from build123d import *

# Parameters (mm, degrees)
ESQUISSE2_W                  = 100
ESQUISSE2_H                  = 100
BOSS_EXTRU_1_DEPTH           = 51
BOSS_EXTRU_1_TAPER           = 20
ENL_V_MAT_EXTRU_1_DEPTH      = 140.622233322
ENL_V_MAT_EXTRU_1_DEPTH_BACK = 140.622233322
ESQUISSE3_R                  = 25
ENL_V_MAT_EXTRU_2_DEPTH      = 140.622233322
ENL_V_MAT_EXTRU_2_DEPTH_BACK = 10
ESQUISSE5_R                  = 35
ENL_V_START                  = -10
ESQUISSE6_R                  = 35
ENL_V_MAT_EXTRU_3_DEPTH      = 10
ESQUISSE7_W                  = 50
ESQUISSE7_H                  = 50
ENL_V_MAT_EXTRU_4_DEPTH      = 140.622233322
CONG_1_R                     = 15
ENL_V_MAT_EXTRU_8_DEPTH      = 10
BOSS_EXTRU_2_DEPTH           = 10
CONG_2_R                     = 5


with BuildPart() as part:
    # Esquisse2 → Boss.-Extru.1 (new body)
    with BuildSketch(Plane.XY):
        with Locations((-23.410404624, -10.838150289)):
            Rectangle(ESQUISSE2_W, ESQUISSE2_H)
    boss_extru_1 = extrude(amount=BOSS_EXTRU_1_DEPTH, taper=BOSS_EXTRU_1_TAPER)

    # Symétrie4: Boss.-Extru.1 across plane
    add(boss_extru_1.mirror(Plane.XY.offset(51)))

    # Esquisse3 → Enlèv. mat.-Extru.1 (cut, two sides: drawn at the far end of the back side and taken through both)
    with BuildSketch(Plane.XY.offset(102).offset(-ENL_V_MAT_EXTRU_1_DEPTH_BACK)):
        with Locations((-23.410404624, -10.838150289)):
            Circle(ESQUISSE3_R)
    extrude(amount=ENL_V_MAT_EXTRU_1_DEPTH + ENL_V_MAT_EXTRU_1_DEPTH_BACK, mode=Mode.SUBTRACT)

    # Esquisse5 → Enlèv. mat.-Extru.2 (cut, two sides: drawn at the far end of the back side and taken through both)
    with BuildSketch(Plane.XY.offset(102).offset(-ENL_V_MAT_EXTRU_2_DEPTH_BACK)):
        with Locations(Location((-23.410404624, -10.838150289, 0), (0, 0, 180))):
            Circle(ESQUISSE5_R)
    extrude(amount=ENL_V_MAT_EXTRU_2_DEPTH + ENL_V_MAT_EXTRU_2_DEPTH_BACK, mode=Mode.SUBTRACT)

    # Esquisse6 → Enlèv. mat.-Extru.3 (cut)
    with BuildSketch(Plane(origin=(0, 0, 0), x_dir=(-1, 0, 0), z_dir=(0, 0, -1)).offset(ENL_V_START)):
        with Locations((23.410404624, -10.838150289)):
            Circle(ESQUISSE6_R)
    extrude(amount=ENL_V_MAT_EXTRU_3_DEPTH, mode=Mode.SUBTRACT)

    # Esquisse7 → Enlèv. mat.-Extru.4 (cut, through all)
    with BuildSketch(Plane(origin=(0, 0, 0), x_dir=(-1, 0, 0), z_dir=(0, 0, -1))):
        with Locations((48.410404624, -35.838150289)):
            Rectangle(ESQUISSE7_W, ESQUISSE7_H)
    extrude(amount=-ENL_V_MAT_EXTRU_4_DEPTH, mode=Mode.SUBTRACT)

    # Congé1
    cong_1_edges = [part.edges().sort_by_distance(p)[0] for p in [
        (8.027113428, -10.838150289, 51),
        (-23.410404624, 20.599367763, 51),
        (-54.847922677, 4.880608737, 51),
    ]]
    fillet(cong_1_edges, radius=CONG_1_R)

    # Esquisse8 → Enlèv. mat.-Extru.8 (cut)
    with BuildSketch(Plane(origin=(0, 0, 0), x_dir=(-1, 0, 0), z_dir=(0, 0, -1))):
        with BuildLine():
            Line((-15.12691495, 31.941809973), (-4.520313233, 21.335208255))
            ThreePointArc((-4.520313233, 21.335208255), (-4.520313233, 17.092567568), (-8.76295392, 17.092567568))
            Line((-8.76295392, 17.092567568), (-19.369555638, 27.699169286))
            ThreePointArc((-19.369555638, 27.699169286), (-19.369555638, 31.941809973), (-15.12691495, 31.941809973))
        make_face()
        with BuildLine():
            Line((-19.369555638, -49.375469864), (-8.76295392, -38.768868146))
            ThreePointArc((-8.76295392, -38.768868146), (-4.520313233, -38.768868146), (-4.520313233, -43.011508833))
            Line((-4.520313233, -43.011508833), (-15.12691495, -53.618110551))
            ThreePointArc((-15.12691495, -53.618110551), (-19.369555638, -53.618110551), (-19.369555638, -49.375469864))
        make_face()
        with BuildLine():
            Line((51.341122481, 21.335208255), (61.947724199, 31.941809973))
            ThreePointArc((61.947724199, 31.941809973), (66.190364886, 31.941809973), (66.190364886, 27.699169286))
            Line((66.190364886, 27.699169286), (55.583763168, 17.092567568))
            ThreePointArc((55.583763168, 17.092567568), (51.341122481, 17.092567568), (51.341122481, 21.335208255))
        make_face()
    extrude(amount=-ENL_V_MAT_EXTRU_8_DEPTH, mode=Mode.SUBTRACT)

    # Esquisse9 → Boss.-Extru.2 (add)
    with BuildSketch(Plane(origin=(0, 0, 0), x_dir=(-1, 0, 0), z_dir=(0, 0, -1))):
        Polygon((-26.589595376, -60.838150289), (23.410404624, -60.838150289), (23.410404624, -57.838150289), (-23.589595376, -57.838150289), (-23.589595376, 36.161849711), (70.410404624, 36.161849711), (70.410404624, -10.838150289), (73.410404624, -10.838150289), (73.410404624, 39.161849711), (-26.589595376, 39.161849711), align=None)
    extrude(amount=BOSS_EXTRU_2_DEPTH)

    # Congé2
    cong_2_edges = [part.edges().sort_by_distance(p)[0] for p in [
        (-23.410404624, 39.161849711, 0),
        (26.589595376, -10.838150289, 0),
        (-73.410404624, 14.161849711, 0),
        (1.589595376, -60.838150289, 0),
    ]]
    fillet(cong_2_edges, radius=CONG_2_R)


solid = part.part
Part model, mm, in its own coordinate system. A direction names the side the tool comes from. Round coordinates to 2 decimals unless told otherwise and drop trailing zeros. Write each loop counter-clockwise with the first axis right and the second up, starting at its lowest first coordinate (ties: lowest second). Pieces come first, ordered by that corner, then holes. Notation, with made-up numbers: M 59.5,12 L 116.5,12 A6 cw 116.5,21 Z; hole C 59.25,33 d1. An arc over 180 degrees is marked long. Return JSON: item names as keys, results as strings. Group by question number.
(1) Pin check, flat tips, straight feed: pin 1 Ø18.5 at (x, y) = (-58.5, 25) entering from -Z; pin 2 Ø5 at (y, z) = (-29, 2) entering from +X (3 decimals); pin 3 Ø2 at (y, z) = (8.5, 85.5) entering from +X. Stop position of each tip, or through.
(2) Saw through at A-A on y = -51. Write the cut outline in (x, z), then the cut area to 3 significant figures.
(3) Saw through at C-C on z = 8.5. Write the cut outline in (x, y).
(4) Two-plate mould, pull along X, no slides. Class faces 1 (the face through (-5.16, 6.25, 50.43)), 2 (the face through (18.36, -10.14, 79.39)), 3 (the face through (-24.11, 30.78, 23.03)): +X half, -X half, draft (parallel to the pull), parting line (faces both ways), or undercut.
(5) Which spindle directions (+Z, -Z, +X, -X, +Y, -Y) get a long thin tool onto all of the face, cutting with end or side? Do faces 4 (the face through (-70.41, 13, -5)), 5 (the face through (14.141, -44.146, 4.93)), 6 (the face through (-65.18, 8.26, 79.39)), 7 (the face through (-24.11, 30.931, 79.386)). Say none if no direction does.
(6) Drill centre lines: probe 1 along Z at (x, y) = (-40, 10); probe 2 along X at (y, z) = (5, 36); probe 3 along Y at (x, z) = (-31.5, -2.5). Where is each one in solid material? Low to high.
(7) Saw through at B-B on x = -10. Write the cut outline in (y, z).
Returned:
{
 "1": {"pin 1": "z = 0", "pin 2": "x = 26.575", "pin 3": "x = 20.95"},
 "2": {"outline": "M -23.41,0 L 12.51,0 L 12.51,10 L 20.21,10 L 20.21,0 L 23.59,0 L 23.59,-10 L 26.59,-10 L 26.59,-0.88 A5 ccw 26.29,0.83 L 16.75,27.03 L -23.41,27.03 Z; M -23.41,74.97 L 16.75,74.97 L 26.59,102 L -23.41,102 Z", "area": "2,390 mm²"},
 "3": {"outline": "M -70.32,-10.84 L -58.41,-10.84 A35 cw long -23.41,-45.84 L -23.41,-57.74 L 23.5,-57.74 L 23.5,36.07 L -70.32,36.07 Z; hole M -66.19,27.7 L -55.58,17.09 A3 ccw -51.34,21.34 L -61.95,31.94 A3 ccw Z; hole M 4.52,-43.01 L 15.13,-53.62 A3 ccw 19.37,-49.38 L 8.76,-38.77 A3 ccw Z; hole M 4.52,21.34 A3 ccw 8.76,17.09 L 19.37,27.7 A3 ccw 15.13,31.94 Z"},
 "4": {"face 1": "undercut", "face 2": "+X half", "face 3": "draft"},
 "5": {"face 4": "-Z, -Y", "face 5": "-Z", "face 6": "-X, +Y, -Y", "face 7": "+X, -X, +Y"},
 "6": {"probe 1": "10 to 92", "probe 2": "-60.31 to -42.75, -4.07 to 13.49", "probe 3": "36.16 to 39.16"},
 "7": {"outline": "M -60.84,-10 L -57.84,-10 L -57.84,0 L -43.17,0 L -43.17,10 L -31.94,10 L -31.94,92 L -43.17,92 L -43.17,102 L -60.84,102 L -42.28,51 L -60.54,0.83 A5 ccw -60.84,-0.88 Z; M 10.26,10 L 21.49,10 L 21.49,0 L 36.16,0 L 36.16,-10 L 39.16,-10 L 39.16,-0.88 A5 ccw 38.86,0.83 L 22.47,45.87 A15 cw 22.47,56.13 L 39.16,102 L 21.49,102 L 21.49,92 L 10.26,92 Z"}
}
